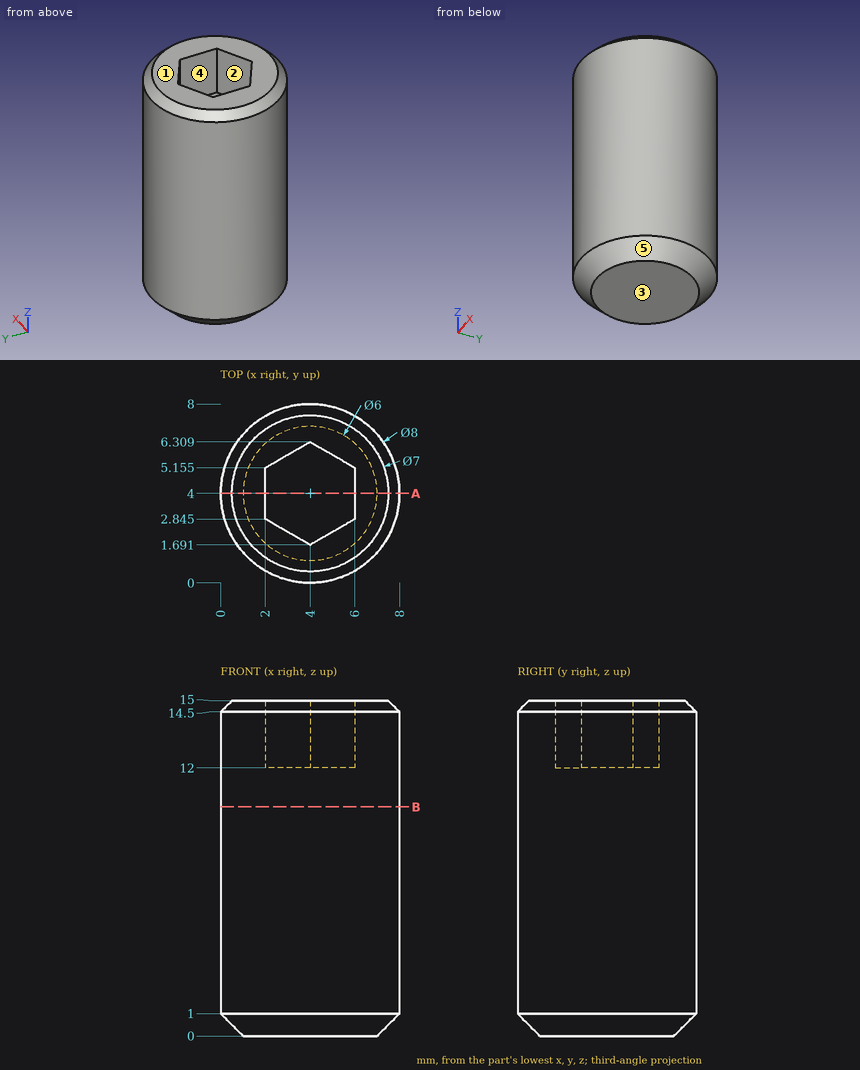
Source: three-view drawing plus pictorial views. Frame: mm from the lowest corner of the part. A direction names the side the tool comes from. Give positions to 0.01 mm unless a question says otherwise; leave off trailing zeros. Loops run counter-clockwise (first coordinate to the right, second up) from the corner with the lowest first, then second, coordinate; pieces in that order, holes last. Notation, with made-up numbers: (-27.5, -26.5) -> (-21.5, -26.5) arc R16 cw to (-21.5, 1.5) -> close; hole circle Ø11 at (47.25, 64.25). An arc over 180 degrees is marked (long way). Use a Markdown table: item, result. Add a question column.
(1) Section query B-B (z = 10.25). Output: boundary loops of the cut face in (x, y).
(2) Access query for the marked faces 1 and 2. Directions: +Z, -Z, +X, -X, +Y, -Y. A direction counts if a zero-diameter tool reaches every point of the face in a straight line with its end or side. Return the directions, or none.
(3) Pull-direction query (Y, two-part tool) for the marked faces 3, 4 and 5; classes: +Y half, -Y half, draft (parallel to the pull), parting line (faces both ways), or undercut.
(4) First-contact query: pin 1 Ø2 at (x, y) = (4, 4.5) entering from +Z. Flat tip, straight axial feed; report the tip coordinate or a pass-through.
(5) Ray query, line 1 (Z direction, x = 3.25, y = 4.5); line 2 (Y direction, x = 2.75, z = 13.5); line 3 (Y direction, x = 7, z = 1.5) (1 decimal). Return the intervals inside material, ascending.
(6) Section query A-A (y = 4). Output: boundary loops of the cut face in (x, z).
Checked values:
| question | item | result |
|---|---|---|
| 1 | outline | circle Ø8 at (4, 4) |
| 2 | face 1 | +Z, +X, -X, +Y, -Y |
| 2 | face 2 | +Z |
| 3 | face 3 | draft |
| 3 | face 4 | undercut |
| 3 | face 5 | parting line |
| 4 | pin 1 | z = 12 |
| 5 | line 1 | 0 to 12 |
| 5 | line 2 | 0.2 to 2.41, 5.59 to 7.8 |
| 5 | line 3 | 1.4 to 6.6 |
| 6 | outline | (0, 1) -> (1, 0) -> (7, 0) -> (8, 1) -> (8, 14.5) -> (7.5, 15) -> (6, 15) -> (6, 12) -> (2, 12) -> (2, 15) -> (0.5, 15) -> (0, 14.5) -> close |
